```python
from build123d import *

# Parameters (mm, degrees)
SKETCH1_W            = 71.12
SKETCH1_H            = 71.12
SKETCH1_R            = 17.78
BOSS_EXTRUDE1_DEPTH  = 0.9525
FILLET1_R            = 8.89
M3_CLEARANCE_HOLE1_D = 3.4


with BuildPart() as part:
    # Sketch1 → Boss-Extrude1 (new body)
    with BuildSketch(Plane(origin=(0, 0, 0), x_dir=(1, 0, 0), z_dir=(0, 1, 0))):
        Rectangle(SKETCH1_W, SKETCH1_H)
        with Locations(Location((0, 0, 0), (0, 0, 90))):
            Circle(SKETCH1_R, mode=Mode.SUBTRACT)
    extrude(amount=BOSS_EXTRUDE1_DEPTH)

    # Fillet1
    fillet1_edges = [part.edges().sort_by_distance(p)[0] for p in [
        (35.56, 0.47625, 35.56),
        (-35.56, 0.47625, 35.56),
        (-35.56, 0.47625, -35.56),
        (35.56, 0.47625, -35.56),
    ]]
    fillet(fillet1_edges, radius=FILLET1_R)

    # M3 Clearance Hole1 (through all)
    with Locations(Plane(origin=(0, 0.9525, 0), x_dir=(1, 0, 0), z_dir=(0, 1, 0))):
        with Locations((-29.21, -29.21), (29.21, -29.21), (29.21, 29.21), (-29.21, 29.21)):
            Hole(M3_CLEARANCE_HOLE1_D / 2)


solid = part.part
```
Build history of the part. All positions in model axes, mm. Give positions to 0.01 mm unless a question says otherwise; leave off trailing zeros. Loops run counter-clockwise (first coordinate to the right, second up) from the corner with the lowest first, then second, coordinate; pieces in that order, holes last. Notation, with made-up numbers: (11.5, -10.5) - (42.5, -10.5) arc R21 ccw to (42.5, 23.5) - close; hole circle Ø4 at (-14, -9). An arc over 180 degrees is marked (long way). Use a Markdown table: item, result.
(1) Drop a flat-ended pin along its axis: pin 1 Ø5 at (x, z) = (11.5, 6.5) entering from -Y. Give the stop position or say it passes through.
Taken from the geometry:
| item | result |
|---|---|
| pin 1 | through |
(2) Band-saw the part on C-C (x = -29.21). Give the cut face in (y, z), and give its area (3 significant figures).
Taken from the geometry:
| item | result |
|---|---|
| outline | (0, -35.19) - (0.95, -35.19) - (0.95, -30.91) - (0, -30.91) - close; (0, -27.51) - (0.95, -27.51) - (0.95, 27.51) - (0, 27.51) - close; (0, 30.91) - (0.95, 30.91) - (0.95, 35.19) - (0, 35.19) - close |
| area | 60.6 mm2 |
(3) Band-saw the part on B-B (z = 0). Give the cut face in (x, y).
Taken from the geometry:
| item | result |
|---|---|
| outline | (-35.56, 0) - (-17.78, 0) - (-17.78, 0.95) - (-35.56, 0.95) - close; (17.78, 0) - (35.56, 0) - (35.56, 0.95) - (17.78, 0.95) - close |
(4) Band-saw the part on A-A (x = 0). Give the cut face in (y, z).
Taken from the geometry:
| item | result |
|---|---|
| outline | (0, -35.56) - (0.95, -35.56) - (0.95, -17.78) - (0, -17.78) - close; (0, 17.78) - (0.95, 17.78) - (0.95, 35.56) - (0, 35.56) - close |
(5) Band-saw the part on D-D (y = 0.6). Give the cut face in (x, z), and give its area (3 significant figures).
Taken from the geometry:
| item | result |
|---|---|
| outline | (-35.56, -26.67) arc R8.89 ccw to (-26.67, -35.56) - (26.67, -35.56) arc R8.89 ccw to (35.56, -26.67) - (35.56, 26.67) arc R8.89 ccw to (26.67, 35.56) - (-26.67, 35.56) arc R8.89 ccw to (-35.56, 26.67) - close; hole circle Ø3.4 at (-29.21, -29.21); hole circle Ø3.4 at (-29.21, 29.21); hole circle Ø35.56 at (0, 0); hole circle Ø3.4 at (29.21, -29.21); hole circle Ø3.4 at (29.21, 29.21) |
| area | 3,960 mm2 |
(6) Pull direction Z, two halves, no side cores. Call faces 1 (the face through (32.89, 0.48, -33.02)), 2 (the face through (29.4, 0.5, -30.9)), 3 (the face through (32.89, 0.48, 33.02)): +Z half, -Z half, draft (parallel to the pull), parting line (faces both ways), or undercut.
Taken from the geometry:
| item | result |
|---|---|
| face 1 | -Z half |
| face 2 | undercut |
| face 3 | +Z half |
(7) Wall check: line 1 along X through (y, z) = (0.4, -29.21); line 2 along X through (y, z) = (0.75, -11.5); line 3 along Z through (x, y) = (-4, 0.6). Give the ranges that are in metal, low to high.
Taken from the geometry:
| item | result |
|---|---|
| line 1 | -35.19 to -30.91, -27.51 to 27.51, 30.91 to 35.19 |
| line 2 | -35.56 to -13.56, 13.56 to 35.56 |
| line 3 | -35.56 to -17.32, 17.32 to 35.56 |
